Design review of the part built by this model. Coordinates are the model's own, in mm. Face numbers are marked on the shaded views. A direction names the side the tool comes from. Round coordinates to 2 decimals unless told otherwise and drop trailing zeros. Loops run counter-clockwise (first coordinate to the right, second up) from the corner with the lowest first, then second, coordinate; pieces in that order, holes last. Notation, with made-up numbers: M 42.25,33.5 L 64.25,33.5 A18 ccw 64.25,64.5 Z; hole C -33.5,37.5 d8. An arc over 180 degrees is marked long. Answer as CSV lines item,"result". Start each with the question number.
from build123d import *

# Parameters (mm, degrees)
ESQUISSE1_R                  = 2
BOSS_EXTRU_1_DEPTH           = 45
ESQUISSE2_W                  = 75
ESQUISSE2_H                  = 39
ENL_V_MAT_EXTRU_1_DEPTH      = 45
ENL_V_MAT_EXTRU_2_DEPTH      = 3.5
ESQUISSE4_W                  = 20
ESQUISSE4_H                  = 8
BOSS_EXTRU_2_DEPTH           = 15
CONG_1_R                     = 3
ENL_V_MAT_EXTRU_3_DEPTH      = 3.5
ENL_V_MAT_EXTRU_4_DEPTH      = 90.930528743
ENL_V_MAT_EXTRU_4_DEPTH_BACK = 90.930528743
ESQUISSE7_R                  = 2


with BuildPart() as part:
    # Esquisse1 → Boss.-Extru.1 (new body)
    with BuildSketch(Plane(origin=(0, 0, 0), x_dir=(1, 0, 0), z_dir=(0, 1, 0))):
        Polygon((77.5, -2.5), (72.5, 2.5), (67.5, 2.5), (67.5, -0.5), (-7.5, -0.5), (-7.5, -8.5), (74.5, -8.5), (74.5, -2.5), align=None)
        with Locations(Location((63.679491924, -4.5, 0), (0, 0, 90))):
            Circle(ESQUISSE1_R, mode=Mode.SUBTRACT)
        with Locations(Location((23.679491924, -4.5, 0), (0, 0, 90))):
            Circle(ESQUISSE1_R, mode=Mode.SUBTRACT)
    extrude(amount=BOSS_EXTRU_1_DEPTH)

    # Esquisse2 → Enlèv. mat.-Extru.1 (cut)
    with BuildSketch(Plane(origin=(0, 0, 0.5), x_dir=(-1, 0, 0), z_dir=(0, 0, -1))):
        with Locations((-30, 19.5)):
            Rectangle(ESQUISSE2_W, ESQUISSE2_H)
    extrude(amount=-ENL_V_MAT_EXTRU_1_DEPTH, mode=Mode.SUBTRACT)

    # Esquisse3 → Enlèv. mat.-Extru.2 (cut)
    with BuildSketch(Plane.XZ.offset(-39)):
        Polygon((65.679491924, 1.035898385), (61.679491924, 1.035898385), (59.679491924, 4.5), (59.679491924, 8.5), (67.679491924, 8.5), (67.679491924, 4.5), align=None)
        Polygon((25.679491924, 1.035898385), (21.679491924, 1.035898385), (19.679491924, 4.5), (19.679491924, 8.5), (27.679491924, 8.5), (27.679491924, 4.5), align=None)
    extrude(amount=-ENL_V_MAT_EXTRU_2_DEPTH, mode=Mode.SUBTRACT)

    # Esquisse4 → Boss.-Extru.2 (add)
    with BuildSketch(Plane.XZ.offset(-39)):
        with Locations((42.5, 4.5)):
            Rectangle(ESQUISSE4_W, ESQUISSE4_H)
        with Locations((4.5, 4.5)):
            Rectangle(ESQUISSE4_W, ESQUISSE4_H)
    extrude(amount=BOSS_EXTRU_2_DEPTH)

    # Congé1
    # the kernel refuses this fillet: 3 mm, written as the material it adds along each edge
    with BuildSketch(Plane(origin=(52.5, 39, 0.5), x_dir=(1, 0, 0), z_dir=(0, 0, 1)), Plane(origin=(32.5, 39, 8.5), x_dir=(-1, 0, 0), z_dir=(0, 0, -1)), Plane(origin=(14.5, 39, 0.5), x_dir=(1, 0, 0), z_dir=(0, 0, 1))) as cong_1_piece_1:
        with BuildLine():
            CenterArc((CONG_1_R, -CONG_1_R), CONG_1_R, 90, 90)
            Line((0, -CONG_1_R), (0, 0))
            Line((0, 0), (CONG_1_R, 0))
        make_face()
    extrude(amount=8)
    with BuildSketch(Plane(origin=(-5.5, 39, 8.5), x_dir=(-1, 0, 0), z_dir=(0, 0, -1))) as cong_1_piece_2:
        with BuildLine():
            CenterArc((3, -2.828427125), CONG_1_R, 109.471220634, 70.528779366)
            Line((0, -2.828427125), (0, 0))
            Line((0, 0), (2, 0))
        make_face()
    extrude(amount=8)
    # the kernel refuses this fillet: 3 mm, written as the material it takes off along each edge
    with BuildSketch(Plane(origin=(52.5, 24, -7), x_dir=(0, 1, 0), z_dir=(0, 0, 1)), Plane(origin=(14.5, 24, -7), x_dir=(0, 1, 0), z_dir=(0, 0, 1))) as cong_1_2_piece_1:
        with BuildLine():
            CenterArc((CONG_1_R, CONG_1_R), CONG_1_R, 180, 90)
            Line((0, CONG_1_R), (0, 0))
            Line((0, 0), (CONG_1_R, 0))
        make_face()
    extrude(amount=23, mode=Mode.SUBTRACT)
    with BuildSketch(Plane(origin=(32.5, 24, 16), x_dir=(1, 0, 0), z_dir=(0, 0, -1)), Plane(origin=(-5.5, 24, 16), x_dir=(1, 0, 0), z_dir=(0, 0, -1))) as cong_1_2_piece_2:
        with BuildLine():
            CenterArc((CONG_1_R, -CONG_1_R), CONG_1_R, 90, 90)
            Line((0, -CONG_1_R), (0, 0))
            Line((0, 0), (CONG_1_R, 0))
        make_face()
    extrude(amount=23, mode=Mode.SUBTRACT)

    # Esquisse5 → Enlèv. mat.-Extru.3 (cut)
    with BuildSketch(Plane.XY.offset(8.5)):
        Polygon((8.5, 32), (6.5, 28.535898385), (2.5, 28.535898385), (0.5, 32), (2.5, 35.464101615), (6.5, 35.464101615), align=None)
        Polygon((46.5, 32), (44.5, 28.535898385), (40.5, 28.535898385), (38.5, 32), (40.5, 35.464101615), (44.5, 35.464101615), align=None)
    extrude(amount=-ENL_V_MAT_EXTRU_3_DEPTH, mode=Mode.SUBTRACT)

    # Esquisse7 → Enlèv. mat.-Extru.4 (cut, two sides: drawn at the far end of the back side and taken through both)
    with BuildSketch(Plane.XY.offset(5).offset(-ENL_V_MAT_EXTRU_4_DEPTH_BACK)):
        with Locations((4.5, 32)):
            Circle(ESQUISSE7_R)
        with Locations((42.5, 32)):
            Circle(ESQUISSE7_R)
    extrude(amount=ENL_V_MAT_EXTRU_4_DEPTH + ENL_V_MAT_EXTRU_4_DEPTH_BACK, mode=Mode.SUBTRACT)


solid = part.part
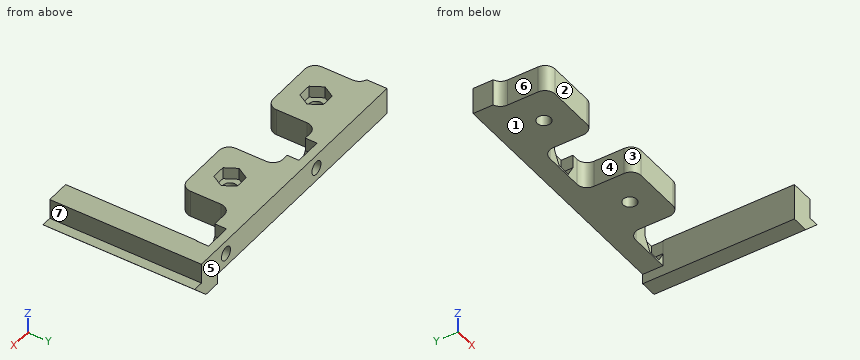
Item 1: Tool access review of the marked faces 1, 2 and 3: name each direction out of +Z, -Z, +X, -X, +Y, -Y from which nothing blocks a thin tool from reaching the whole face with its end or side.
Item 2: To check wall thickness, follow line 1 (X direction, y = 32, z = 6); line 2 (X direction, y = 43.9, z = 4.5); line 3 (X direction, y = 32, z = 2.6). State the ranges of each line that lie inside material, in increasing order.
Item 3: Consider section C-C, the plane x = 5. Write out the cut boundary in (y, z).
Item 4: The part is to be moulded in two halves that separate along X. For the marked faces 4, 5, 6 and 7, say which applies: +X half, -X half, draft (parallel to the pull), parting line (faces both ways), or undercut.
Item 5: Insertion check: pin 1 Ø4 at (y, z) = (19.5, 7) entering from +X; pin 2 Ø2.5 at (y, z) = (29.5, 5.5) entering from -X; pin 3 Ø4 at (x, y) = (1, 34.5) entering from -Z; pin 4 Ø3 at (x, z) = (63.68, 4.5) entering from -Y. Each pin has a flat end and moves straight along its axis. Give the tip position at first contact, or say it passes through.
Item 6: Consider section A-A, the plane x = 42.5. Write out the cut boundary in (y, z).
Item 7: Consider section B-B, the plane y = 7. Write out the cut boundary in (x, z).
Found:
1,face 1,"-Z, -X, +Y, -Y"
1,face 2,"+Z, -Z, -X, -Y"
1,face 3,"+Z, -Z, -Y"
2,line 1,"x = -5.5 to 0.5, 8.5 to 14.5, 32.5 to 38.5, 46.5 to 52.5, 67.5 to 74.5"
2,line 2,"x = -7.5 to 21.68, 25.68 to 61.68, 65.68 to 74.5"
2,line 3,"x = -5.5 to 2.5, 6.5 to 14.5, 32.5 to 40.5, 44.5 to 52.5, 67.5 to 74.5"
3,outline,"M 24,0.5 L 30.06,0.5 L 30.06,5 L 28.54,5 L 28.54,8.5 L 24,8.5 Z; M 33.94,0.5 L 45,0.5 L 45,8.5 L 35.46,8.5 L 35.46,5 L 33.94,5 Z"
4,face 4,"undercut"
4,face 5,"draft"
4,face 6,"-X half"
4,face 7,"+X half"
5,pin 1,"stops at x = 74.5"
5,pin 2,"stops at x = -5.5"
5,pin 3,"stops at z = 0.5"
5,pin 4,"passes through"
6,outline,"M 24,0.5 L 30,0.5 L 30,5 L 28.54,5 L 28.54,8.5 L 24,8.5 Z; M 34,0.5 L 45,0.5 L 45,8.5 L 35.46,8.5 L 35.46,5 L 34,5 Z"
7,outline,"M 67.5,-2.5 L 72.5,-2.5 L 77.5,2.5 L 74.5,2.5 L 74.5,8.5 L 67.5,8.5 Z"
